The listing builds one solid part. Answer for the finished solid, in the listing's coordinates (mm). A direction names the side the tool comes from. Round coordinates to 2 decimals unless told otherwise and drop trailing zeros. Loops run counter-clockwise (first coordinate to the right, second up) from the corner with the lowest first, then second, coordinate; pieces in that order, holes last. Notation, with made-up numbers: (86.5, 48) - (143.5, 48) arc R21 cw to (143.5, 54) - close; hole circle Ø9 at (39, -37). An arc over 180 degrees is marked (long way). One line per item, written item: value.
```python
from build123d import *

# Parameters (mm, degrees)
BOSS_EXTRUDE1_DEPTH     = 8
SKETCH2_R               = 1.5
CUT_EXTRUDE1_DEPTH      = 5.9
CUT_EXTRUDE1_DEPTH_BACK = 4.4
CUT_EXTRUDE2_START      = 4.9
SKETCH2_3_R             = 1.5
CUT_EXTRUDE2_DEPTH      = 1
SKETCH3_R               = 3
CUT_EXTRUDE3_DEPTH      = 1
FILLET1_R               = 4


with BuildPart() as part:
    # Sketch1 → Boss-Extrude1 (new body)
    with BuildSketch(Plane(origin=(0, 0, 0), x_dir=(1, 0, 0), z_dir=(0, 1, 0))):
        with BuildLine():
            Line((-8.65, -0.75), (-8.65, -4.15))
            Line((-8.65, -4.15), (4.15, -4.15))
            Line((4.15, -4.15), (4.15, 4.15))
            Line((4.15, 4.15), (-8.65, 4.15))
            Line((-8.65, 4.15), (-8.65, 0.75))
            Line((-8.65, 0.75), (-2.014944168, 0.75))
            ThreePointArc((-2.014944168, 0.75), (0.38103152, 2.115966678), (2.15, 0))
            ThreePointArc((2.15, 0), (0.38103152, -2.115966678), (-2.014944168, -0.75))
            Line((-2.014944168, -0.75), (-8.65, -0.75))
        make_face()
    extrude(amount=BOSS_EXTRUDE1_DEPTH)

    # Sketch2 → Cut-Extrude1 (cut, two sides)
    with BuildSketch(Plane.XY.offset(-0.75)) as cut_extrude1_sk:
        with Locations((-4.014944168, 4)):
            Circle(SKETCH2_R)
    extrude(amount=CUT_EXTRUDE1_DEPTH, mode=Mode.SUBTRACT)
    extrude(cut_extrude1_sk.sketch, amount=-CUT_EXTRUDE1_DEPTH_BACK, mode=Mode.SUBTRACT)

    # Sketch2<3> → Cut-Extrude2 (cut)
    with BuildSketch(Plane.XY.offset(-0.75).offset(CUT_EXTRUDE2_START)):
        Polygon((-2.014944168, 6.309401077), (-4.014944168, 7.464101615), (-7.014944168, 5.732050808), (-7.014944168, 2.267949192), (-4.014944168, 0.535898385), (-2.014944168, 1.690598923), align=None)
        with Locations((-4.014944168, 4)):
            Circle(SKETCH2_3_R, mode=Mode.SUBTRACT)
        Polygon((-1.014944168, 5.732050808), (-2.014944168, 6.309401077), (-2.014944168, 1.690598923), (-1.014944168, 2.267949192), align=None)
    extrude(amount=-CUT_EXTRUDE2_DEPTH, mode=Mode.SUBTRACT)

    # Sketch3 → Cut-Extrude3 (cut)
    with BuildSketch(Plane(origin=(0, 0, -4.15), x_dir=(-1, 0, 0), z_dir=(0, 0, -1))):
        with Locations((4.014944168, 4)):
            Circle(SKETCH3_R)
    extrude(amount=-CUT_EXTRUDE3_DEPTH, mode=Mode.SUBTRACT)

    # Fillet1
    fillet1_edges = [part.edges().sort_by_distance(p)[0] for p in [
        (4.15, 4, -4.15),
        (4.15, 4, 4.15),
    ]]
    fillet(fillet1_edges, radius=FILLET1_R)


solid = part.part
```
1) A cutting plane is placed at C-C on z = 1.25. Give the vertices of the cut face in (x, y).
Final values:
outline: (-8.65, 0) - (-1.75, 0) - (-1.75, 8) - (-8.65, 8) - close; (1.75, 0) - (4, 0) - (4, 8) - (1.75, 8) - close; hole circle Ø3 at (-4.01, 4)
2) Consider L1, parallel to X at y = 3.5, z = 1.75; L2, parallel to Y at x = -3.5, z = 3; L3, parallel to Z at x = -1.25, y = 7.75. Determine where each line is inside the solid, lowest interval first.
Final values:
L1: -8.65 to -5.43, -2.6 to -1.25, 1.25 to 3.82
L2: 0 to 2.59, 5.41 to 8
L3: -4.15 to -1.75, 1.75 to 4.15
3) A cutting plane is placed at D-D on x = 1. Give the vertices of the cut face in (y, z).
Final values:
outline: (0, -4.06) - (8, -4.06) - (8, -1.9) - (0, -1.9) - close; (0, 1.9) - (8, 1.9) - (8, 4.06) - (0, 4.06) - close
4) A cutting plane is placed at B-B on x = -3.25. Give the vertices of the cut face in (y, z), and give its area (3 significant figures).
Final values:
outline: (0, -4.15) - (1.1, -4.15) - (1.1, -3.15) - (2.71, -3.15) - (2.71, -0.75) - (0, -0.75) - close; (0, 0.75) - (2.71, 0.75) - (2.71, 3.15) - (0.98, 3.15) - (0.98, 4.15) - (0, 4.15) - close; (5.29, -3.15) - (6.9, -3.15) - (6.9, -4.15) - (8, -4.15) - (8, -0.75) - (5.29, -0.75) - close; (5.29, 0.75) - (8, 0.75) - (8, 4.15) - (7.02, 4.15) - (7.02, 3.15) - (5.29, 3.15) - close
area: 30.2 mm2
5) Each of these flat-tipped pins is pushed along its axis until it touches: pin 1 Ø3 at (x, y) = (-3.5, 3.5) entering from -Z; pin 2 Ø4 at (x, z) = (1, 1.5) entering from -Y; pin 3 Ø4 at (x, y) = (-4.01, 4) entering from +Z; pin 4 Ø1.1 at (y, z) = (4.5, 3.5) entering from +X. Where does it stop, or does it pass through?
Final values:
pin 1: z = -3.15
pin 2: y = 0
pin 3: z = 3.15
pin 4: x = 3.01
6) A cutting plane is placed at A-A on y = 4. Give the vertices of the cut face in (x, z), and give its area (3 significant figures).
Final values:
outline: (-8.65, -4.15) - (-7.01, -4.15) - (-7.01, -3.15) - (-5.51, -3.15) - (-5.51, -0.75) - (-8.65, -0.75) - close; (-8.65, 0.75) - (-5.51, 0.75) - (-5.51, 3.15) - (-7.01, 3.15) - (-7.01, 4.15) - (-8.65, 4.15) - close; (-2.51, -3.15) - (-1.01, -3.15) - (-1.01, -4.15) - (0.15, -4.15) arc R4 ccw to (4.15, -0.15) - (4.15, 0.15) arc R4 ccw to (0.15, 4.15) - (-1.01, 4.15) - (-1.01, 3.15) - (-2.51, 3.15) - (-2.51, 0.75) - (-2.01, 0.75) arc R2.15 cw (long way) to (-2.01, -0.75) - (-2.51, -0.75) - close
area: 48.6 mm2
7) For faces 1 (the flat face through (-6, 4, 0.75)), 2 (the cylindrical face through (-1.634, 2.175, -3.657)), 3 (the flat face through (-4, 0, 1)), 4 (the flat face through (-2.536, 1.39, 3.657)), determine the directions among +Z, -Z, +X, -X, +Y, -Y from which every point of the face is accessible in a straight line to the end or side of a thin tool.
Final values:
face 1: -X, +Y, -Y
face 2: -Z
face 3: +Z, -Z, +X, -X, -Y
face 4: +Z
8) For a pull along Z with two mould halves and no side action, classify faces 5 (the flat face through (-6, 4, -0.75)), 6 (the flat face through (-4.724, 2.509, 3.15)), 7 (the cylindrical face through (-3.209, 5.265, -1.933)), 8 (the cylindrical face through (3.009, 4.056, -2.947)) as released by +Z, released by -Z, zero draft, split by the parting line, or undercut.
Final values:
face 5: undercut
face 6: released by +Z
face 7: zero draft
face 8: released by -Z
